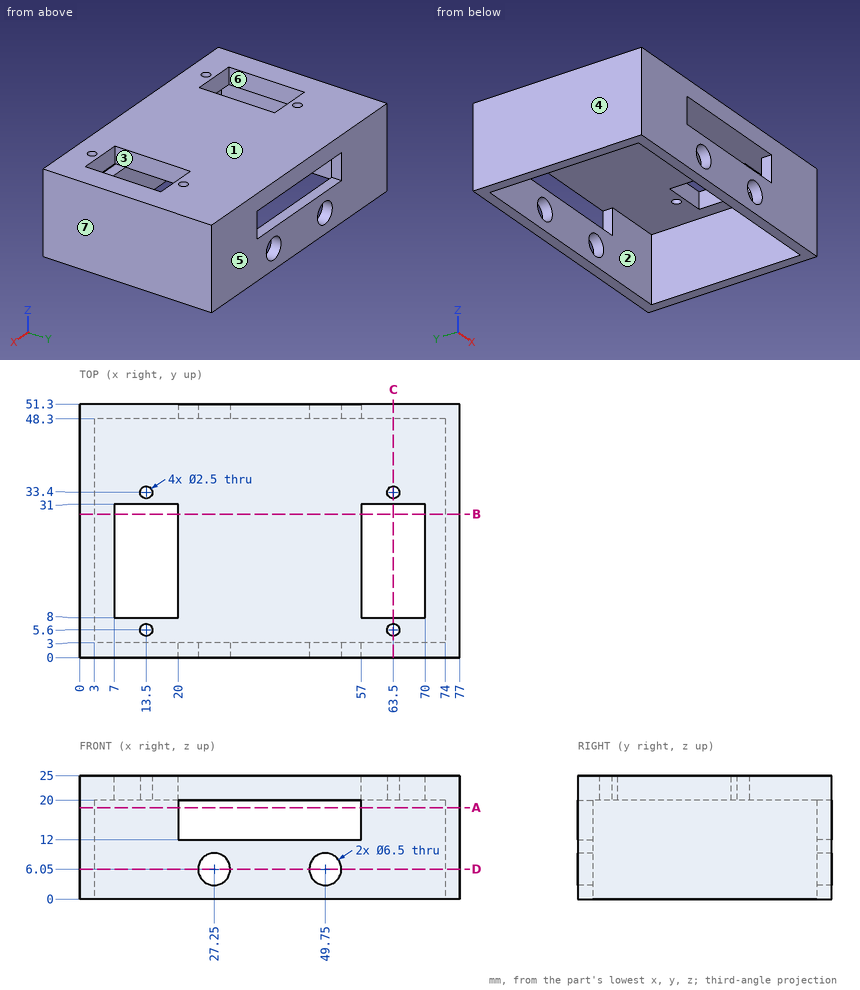
Source: three-view drawing plus pictorial views. Frame: mm from the lowest corner of the part. A direction names the side the tool comes from. Give positions to 0.01 mm unless a question says otherwise; leave off trailing zeros. Loops run counter-clockwise (first coordinate to the right, second up) from the corner with the lowest first, then second, coordinate; pieces in that order, holes last. Notation, with made-up numbers: (3.5, 73.5) -> (22.5, 73.5) arc R21 ccw to (22.5, 91.5) -> close; hole circle Ø1 at (-11.5, -33). An arc over 180 degrees is marked (long way). Put each result on its own line as item: value. Start each with the question number.
1) Reachability of the marked faces 1, 2 and 3 from +Z, -Z, +X, -X, +Y, -Y: full face, straight path, thin tool, end or side. Return the list, or none.
2) Material intervals for probe 1 along Z at (x, y) = (27.25, 1.55); probe 2 along X at (y, z) = (5.6, 21.4); probe 3 along X at (y, z) = (9, 19.5), sorted ascending.
3) Contact query for flat-ended pins moving along their axis: P1, Ø3, axis at x = 63.5, y = 33.4, coming from the -Z side; P2, Ø2, axis at x = 13.5, y = 33.4, coming from the +Z side. Output: stop coordinate, or through.
4) Cut plane A-A (z = 18.5). Return loops of the section in (x, y).
5) Cut plane B-B (y = 29). Return loops of the section in (x, z), then the cut area to 3 significant figures.
6) Draft query along X for the marked faces 4, 5, 6 and 7. Return one class per face: released by +X, released by -X, zero draft, split by the parting line, or undercut.
7) Cut plane D-D (z = 6.05). Return loops of the section in (x, y), then the cut area to 3 significant figures.
8) Cut plane C-C (x = 63.5). Return loops of the section in (y, z).
Results are:
1. face 1: +Z, +X, -X, +Y, -Y
1. face 2: -Z
1. face 3: +Z, -Z
2. probe 1: z = 0 to 2.8, 9.3 to 12, 20 to 25
2. probe 2: x = 0 to 12.25, 14.75 to 62.25, 64.75 to 77
2. probe 3: x = 0 to 3, 74 to 77
3. P1: stops at z = 20
3. P2: passes through
4. outline: (0, 0) -> (20, 0) -> (20, 3) -> (3, 3) -> (3, 48.3) -> (20, 48.3) -> (20, 51.3) -> (0, 51.3) -> close; (57, 0) -> (77, 0) -> (77, 51.3) -> (57, 51.3) -> (57, 48.3) -> (74, 48.3) -> (74, 3) -> (57, 3) -> close
5. outline: (0, 0) -> (3, 0) -> (3, 20) -> (7, 20) -> (7, 25) -> (0, 25) -> close; (20, 20) -> (57, 20) -> (57, 25) -> (20, 25) -> close; (70, 20) -> (74, 20) -> (74, 0) -> (77, 0) -> (77, 25) -> (70, 25) -> close
5. area: 375 mm2
6. face 4: released by -X
6. face 5: zero draft
6. face 6: undercut
6. face 7: released by +X
7. outline: (0, 0) -> (24, 0) -> (24, 3) -> (3, 3) -> (3, 48.3) -> (24, 48.3) -> (24, 51.3) -> (0, 51.3) -> close; (30.5, 0) -> (46.5, 0) -> (46.5, 3) -> (30.5, 3) -> close; (30.5, 48.3) -> (46.5, 48.3) -> (46.5, 51.3) -> (30.5, 51.3) -> close; (53, 0) -> (77, 0) -> (77, 51.3) -> (53, 51.3) -> (53, 48.3) -> (74, 48.3) -> (74, 3) -> (53, 3) -> close
7. area: 656 mm2
8. outline: (0, 0) -> (3, 0) -> (3, 20) -> (4.35, 20) -> (4.35, 25) -> (0, 25) -> close; (6.85, 20) -> (8, 20) -> (8, 25) -> (6.85, 25) -> close; (31, 20) -> (32.15, 20) -> (32.15, 25) -> (31, 25) -> close; (34.65, 20) -> (48.3, 20) -> (48.3, 0) -> (51.3, 0) -> (51.3, 25) -> (34.65, 25) -> close
